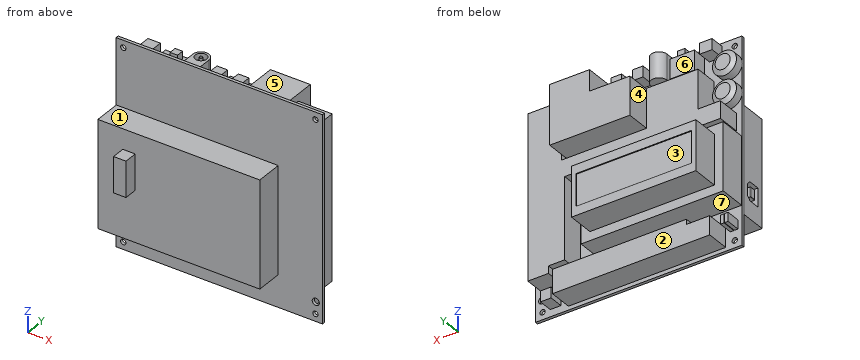
```python
from build123d import *
from OCP.BRepFilletAPI import BRepFilletAPI_MakeChamfer

# Parameters (mm, degrees)
SKETCH1_W              = 116
SKETCH1_H              = 115
SKETCH1_R              = 1.5
BASE_FLANGE1_DEPTH     = 1.65
SKETCH3_W              = 79.9
SKETCH3_H              = 38
EXTRUDE1_DEPTH         = 15
SKETCH4_W              = 69.9
SKETCH4_H              = 28
EXTRUDE2_DEPTH         = 15
SKETCH6_W              = 64.9
SKETCH6_H              = 18
DISPLAY_DEPTH          = 0.53
SKETCH7_W              = 91
SKETCH7_H              = 60
WIRING_BOARD_DEPTH     = 15
SKETCH8_W              = 7
SKETCH8_H              = 20
EXTRUDE5_DEPTH         = 7.5
SKETCH9_W              = 10.5
SKETCH9_H              = 8.5
SKETCH9_W_2            = 5.5
SKETCH9_H_2            = 3.5
USB_DEPTH              = 7.5
CHAMFER1_SIZE          = 2
SKETCH10_R             = 6.75
POTENTIOMETERS_DEPTH   = 6.2
SKETCH11_W             = 7
SKETCH11_H             = 6.1
SKETCH11_W_2           = 9
SKETCH11_H_2           = 14.3
SKETCH11_W_3           = 6
SKETCH11_H_3           = 6
SKETCH11_W_4           = 2
SKETCH11_H_4           = 5
KEEP_ACCESSIBLE_DEPTH  = 8
EXTRUDE9_DEPTH         = 13
HOT_VOLTAGE_REGS_DEPTH = 23.5
SKETCH14_R             = 4.5
EXTRUDE10_DEPTH        = 14.3
EXTRUDE11_DEPTH        = 10
EXTRUDE11_DEPTH_BACK   = 3.4
SKETCH15_R             = 3.219788924
SKETCH15_R_2           = 0.896300673
SKETCH15_W             = 5.949829442
SKETCH15_H             = 2.638553101
SKETCH15_H_2           = 2.133019186
FILLET1_R              = 0.2
CHAMFER2_SIZE          = 1.5
CHAMFER2_SIZE2         = 2.5
SKETCH16_R             = 2
EXTRUDE12_DEPTH        = 10


# Sheet-metal steps are written as plain solids
with BuildPart() as part:
    # Sketch1 → Base-Flange1 (new body)
    with BuildSketch(Plane(origin=(0, 0, 0), x_dir=(1, 0, 0), z_dir=(0, 1, 0))):
        Rectangle(SKETCH1_W, SKETCH1_H)
        with Locations(Location((54, 53.4, 0), (0, 0, 270))):
            Circle(SKETCH1_R, mode=Mode.SUBTRACT)
        with Locations(Location((54, -53.4, 0), (0, 0, 90))):
            Circle(SKETCH1_R, mode=Mode.SUBTRACT)
        with Locations(Location((-54, 53.4, 0), (0, 0, 90))):
            Circle(SKETCH1_R, mode=Mode.SUBTRACT)
        with Locations(Location((-54, -53.4, 0), (0, 0, 270))):
            Circle(SKETCH1_R, mode=Mode.SUBTRACT)
    extrude(amount=BASE_FLANGE1_DEPTH)

    # Sketch3 → Extrude1 (add)
    with BuildSketch(Plane(origin=(0, 1.65, 0), x_dir=(1, 0, 0), z_dir=(0, 1, 0))):
        with Locations((-17.95, 16.5)):
            Rectangle(SKETCH3_W, SKETCH3_H)
    extrude(amount=EXTRUDE1_DEPTH)

    # Sketch4 → Extrude2 (add)
    with BuildSketch(Plane(origin=(0, 16.65, 0), x_dir=(1, 0, 0), z_dir=(0, 1, 0))):
        with Locations((-17.95, 16.5)):
            Rectangle(SKETCH4_W, SKETCH4_H)
    extrude(amount=EXTRUDE2_DEPTH)

    # Sketch6 → Display! (cut)
    with BuildSketch(Plane(origin=(0, 31.65, 0), x_dir=(1, 0, 0), z_dir=(0, 1, 0))):
        with Locations((-17.95, 16.5)):
            Rectangle(SKETCH6_W, SKETCH6_H)
    extrude(amount=-DISPLAY_DEPTH, mode=Mode.SUBTRACT)

    # Sketch7 → Wiring Board (add)
    with BuildSketch(Plane.XZ):
        with Locations((-12.4, -9.5)):
            Rectangle(SKETCH7_W, SKETCH7_H)
    extrude(amount=WIRING_BOARD_DEPTH)

    # Sketch8 → Extrude5 (add)
    with BuildSketch(Plane.XZ.offset(15)):
        with Locations((-40.4, -0.8)):
            Rectangle(SKETCH8_W, SKETCH8_H)
    extrude(amount=EXTRUDE5_DEPTH)

    # Sketch9 → USB (cut)
    with BuildSketch(Plane.ZY.offset(58)):
        with Locations((-24.25, -7.35)):
            Rectangle(SKETCH9_W, SKETCH9_H)
        with Locations((-24.25, -7.35)):
            Rectangle(SKETCH9_W_2, SKETCH9_H_2, mode=Mode.SUBTRACT)
    extrude(amount=-USB_DEPTH, mode=Mode.SUBTRACT)

    # Chamfer1
    chamfer1_edges = [part.edges().sort_by_distance(p)[0] for p in [
        (-54.2, -3.1, -19),
        (-54.2, -3.1, -29.5),
    ]]
    chamfer(chamfer1_edges, length=CHAMFER1_SIZE)

    # Sketch10 → Potentiometers (add)
    with BuildSketch(Plane(origin=(0, 1.65, 0), x_dir=(1, 0, 0), z_dir=(0, 1, 0))):
        with Locations(Location((-51.5, -26.5, 0), (0, 0, 164.357528987))):
            Circle(SKETCH10_R)
        with Locations(Location((-51.5, -42.5, 0), (0, 0, 164.357528987))):
            Circle(SKETCH10_R)
    extrude(amount=POTENTIOMETERS_DEPTH)

    # Sketch11 → Keep Accessible!! (add)
    with BuildSketch(Plane(origin=(0, 1.65, 0), x_dir=(1, 0, 0), z_dir=(0, 1, 0))):
        Polygon((-26.092034571, -53.3), (-23.1, -53.3), (-23.1, -42.3), (-36.9, -42.3), (-36.9, -53.3), (-30.292034571, -53.3), (-30.292034571, -57.5), (-26.092034571, -57.5), align=None)
        with Locations((-43.3, -52.95)):
            Rectangle(SKETCH11_W, SKETCH11_H)
        with Locations((-17, -49.55)):
            Rectangle(SKETCH11_W_2, SKETCH11_H_2)
        with Locations((-5, -52.1)):
            Rectangle(SKETCH11_W_3, SKETCH11_H_3)
        with Locations((7, -52.1)):
            Rectangle(SKETCH11_W_3, SKETCH11_H_3)
        with Locations((46.66, 50.5)):
            Rectangle(SKETCH11_W_3, SKETCH11_H_3)
        with Locations((-54.82, 45.3)):
            Rectangle(SKETCH11_W_4, SKETCH11_H_4)
        with Locations((-52.52, 45.3)):
            Rectangle(SKETCH11_W_4, SKETCH11_H_4)
    extrude(amount=KEEP_ACCESSIBLE_DEPTH)

    # Sketch12 → Extrude9 (add)
    with BuildSketch(Plane(origin=(0, 1.65, 0), x_dir=(1, 0, 0), z_dir=(0, 1, 0))):
        Polygon((-48.948570669, 53.670290093), (-48.948570669, 44.832154672), (-35.833918109, 44.832154672), (-35.833918109, 41.981143246), (37.294524965, 41.981143246), (39.432783534, 41.981143246), (39.432783534, 53.670290093), (39.432783534, 55.380896948), (-48.948570669, 55.380896948), align=None)
        Polygon((41.713592675, 43.406648959), (41.713592675, 39.272682392), (32.590356112, 39.272682392), (32.590356112, -6.486050994), (-54.935694663, -6.486050994), (-54.935694663, -16.179489842), (-42.391244389, -16.179489842), (-42.391244389, -38.132277821), (-13.310927845, -38.132277821), (-13.310927845, -16.179489842), (34.300962968, -16.179489842), (34.300962968, -48.538469526), (53.26018895, -48.538469526), (53.26018895, 43.406648959), align=None)
    extrude(amount=EXTRUDE9_DEPTH)

    # Sketch13 → Hot! Voltage Regs (add)
    with BuildSketch(Plane(origin=(0, 1.65, 0), x_dir=(1, 0, 0), z_dir=(0, 1, 0))):
        Polygon((-11.315219847, -18.602849554), (-11.315219847, -40.12798582), (11.350320989, -40.12798582), (11.350320989, -51.959683237), (33.730760683, -51.959683237), (33.730760683, -18.602849554), align=None)
    extrude(amount=HOT_VOLTAGE_REGS_DEPTH)

    # Sketch14 → Extrude10 (add)
    with BuildSketch(Plane.XY.offset(56.7)):
        with Locations((-17, 9.65)):
            Circle(SKETCH14_R)
    extrude(amount=-EXTRUDE10_DEPTH)

    # Sketch15 → Extrude11 (cut, two sides: drawn at the far end of the back side and taken through both)
    # profile 1 of 3: a face of its own
    with BuildSketch(Plane.XY.offset(56.7).offset(-EXTRUDE11_DEPTH_BACK)):
        with Locations(Location((-17, 9.65, 0), (0, 0, 180))):
            Circle(SKETCH15_R)
        with Locations(Location((-17, 9.65, 0), (0, 0, 180))):
            Circle(SKETCH15_R_2, mode=Mode.SUBTRACT)
    # profile 2 of 3: a face of its own
    with BuildSketch(Plane.XY.offset(56.7).offset(-EXTRUDE11_DEPTH_BACK)):
        with Locations((-28.188847243, 9.227024123)):
            Rectangle(SKETCH15_W, SKETCH15_H)
    # profile 3 of 3: a face of its own
    with BuildSketch(Plane.XY.offset(56.7).offset(-EXTRUDE11_DEPTH_BACK)):
        with Locations((-28.188847243, 2.716509593)):
            Rectangle(SKETCH15_W, SKETCH15_H_2)
    extrude(amount=EXTRUDE11_DEPTH + EXTRUDE11_DEPTH_BACK, mode=Mode.SUBTRACT)

    # Fillet1
    fillet1_edges = [part.edges().sort_by_distance(p)[0] for p in [
        (-16.103699327, 9.65, 56.7),
        (-57.9, -9.1, -24.25),
        (-57.9, -7.35, -21.5),
        (-57.9, -5.6, -24.25),
        (-57.9, -7.35, -27),
    ]]
    fillet(fillet1_edges, radius=FILLET1_R)

    # Chamfer2: one chamfer whose edges measure the first distance from different faces: ONE call of the kernel's chamfer builder (chamfer() names one face for all edges)
    chamfer2_edges_1 = [part.edges().sort_by_distance(p)[0] for p in [
        (-45, 7.85, 28.320027472),
    ]]
    chamfer2_side_1 = [part.faces().sort_by_distance(p)[0] for p in [
        (-45, 4.75, 28.320027472),
    ]]
    chamfer2_edges_2 = [part.edges().sort_by_distance(p)[0] for p in [
        (-45, 7.85, 44.320027472),
    ]]
    chamfer2_side_2 = [part.faces().sort_by_distance(p)[0] for p in [
        (-45, 4.75, 44.320027472),
    ]]
    chamfer2 = BRepFilletAPI_MakeChamfer(part.part.solid().wrapped)
    for e in chamfer2_edges_1:
        chamfer2.Add(CHAMFER2_SIZE, CHAMFER2_SIZE2, e.wrapped, chamfer2_side_1[0].wrapped)  # the first distance lies on this face
    for e in chamfer2_edges_2:
        chamfer2.Add(CHAMFER2_SIZE, CHAMFER2_SIZE2, e.wrapped, chamfer2_side_2[0].wrapped)  # the first distance lies on this face
    add(Compound.cast(chamfer2.Shape()), mode=Mode.REPLACE)

    # Sketch16 → Extrude12 (cut)
    with BuildSketch(Plane(origin=(0, 1.65, 0), x_dir=(1, 0, 0), z_dir=(0, 1, 0))):
        with Locations(Location((54.2, 46.7, 0), (0, 0, 270))):
            Circle(SKETCH16_R)
    extrude(amount=-EXTRUDE12_DEPTH, mode=Mode.SUBTRACT)


solid = part.part
```
Design review of the part built by this model. Coordinates are the model's own, in mm. Face numbers are marked on the shaded views. A direction names the side the tool comes from. Coordinates: 2 decimals unless noted, no trailing zeros. Order: outer loops, then holes, each group sorted by start corner. A loop starts at its lowest first (then second) coordinate and runs counter-clockwise, first axis right, second up.
1) Wall thickness on line 1 along X through (y, z) = (0.65, -53.4); line 2 along Z through (x, y) = (0, 11); line 3 along Z through (x, y) = (-51, -6): over which ranges is each line inside the solid? List them lowest first.
2) For the marked faces 4, 5, 6 and 7, list the 3-axis set-ups (+Z, -Z, +X, -X, +Y, -Y) from which the entire face can be reached by the end or side of a thin tool; tool diameter is ignored.
3) Mouldability with a two-part tool opening along Z and no side actions: class the marked faces 1, 2 and 3 as +Z half, -Z half, draft (parallel to the pull), parting line (faces both ways), or undercut.
4) Take a section at A-A, the plane y = -13.5. Give the boundary of the cut face in (x, z), and give its area (3 significant figures).
5) Clearance check with flat-ended pins moving along their axes: pin 1 (12 mm diameter, centred on x = 5, z = 39.5, fed in from -Y); pin 2 (4.5 mm diameter, centred on x = -2, y = 7.5, fed in from -Z); pin 3 (4 mm diameter, centred on y = -4, z = 14.5, fed in from +X). State where each tip first meets the part, or that it passes through.
Returned:
1. line 1: x = -58 to -55.5, -52.5 to 52.5, 55.5 to 58
1. line 2: z = -55.38 to -41.98, -35.5 to 2.5, 6.49 to 16.18, 18.6 to 40.13
1. line 3: z = -39.5 to -29.5, -27 to -21.5, -19 to 20.5
2. face 4: +Z, +Y
2. face 5: +Z, +X, +Y
2. face 6: +Z, -X, +Y
2. face 7: -X, +Y
3. face 1: +Z half
3. face 2: draft
3. face 3: undercut
4. outline: (-57.9, -39.5) - (33.1, -39.5) - (33.1, 20.5) - (-57.9, 20.5) - close
4. area: 5,460 mm2
5. pin 1: stops at y = 0
5. pin 2: stops at z = -55.38
5. pin 3: stops at x = 33.1
